Design review of the part built by this model. Coordinates are the model's own, in mm. Face numbers are marked on the shaded views. A direction names the side the tool comes from. Coordinates: 2 decimals unless noted, no trailing zeros. Loops run counter-clockwise (first coordinate to the right, second up) from the corner with the lowest first, then second, coordinate; pieces in that order, holes last. Notation, with made-up numbers: M -21.75,-23.75 L 15.25,-23.75 A29 ccw 15.25,11.25 Z; hole C 88.5,36 d9. An arc over 180 degrees is marked long. One line per item, written item: value.
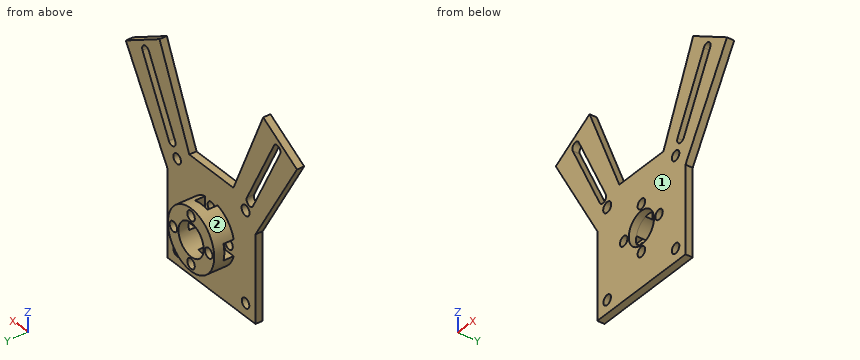
```python
from build123d import *

# Parameters (mm, degrees)
SKETCH_1_R          = 1.7
SKETCH_1_R_2        = 1.8
SKETCH_1_R_3        = 5.7
EXTRUDE_1_DEPTH     = 2.5
SKETCH_2_R          = 10.5
EXTRUDE_2_DEPTH     = 7
SKETCH_4_R          = 1.7
CUT_EXTRUDE_1_DEPTH = 7
CUT_EXTRUDE_2_DEPTH = 3.5
SKETCH_6_R          = 5.7
CUT_EXTRUDE_3_DEPTH = 20


with BuildPart() as part:
    # 草图1 → 凸台-拉伸1 (new body)
    with BuildSketch(Plane(origin=(0, 0, 0), x_dir=(1, 0, 0), z_dir=(0, 1, 0))):
        Polygon((-9.99944515, -20.000324527), (10.00055485, -20.000324527), (23.493176713, -51.085714784), (38.795982487, -42.134997854), (20, -10), (20, 20), (-20, 20), (-20, -10), (-38.79573581, -42.1354119), (-23.493239928, -51.085714784), align=None)
        with Locations((15.5, 15.5)):
            Circle(SKETCH_1_R, mode=Mode.SUBTRACT)
        with Locations((-15.5, -15.5)):
            Circle(SKETCH_1_R_2, mode=Mode.SUBTRACT)
        with Locations((-15.5, 15.5)):
            Circle(SKETCH_1_R, mode=Mode.SUBTRACT)
        Circle(SKETCH_1_R_3, mode=Mode.SUBTRACT)
        with Locations((-8, 0)):
            Circle(SKETCH_1_R, mode=Mode.SUBTRACT)
        with Locations((0, 8)):
            Circle(SKETCH_1_R, mode=Mode.SUBTRACT)
        with Locations((8, 0)):
            Circle(SKETCH_1_R, mode=Mode.SUBTRACT)
        with Locations((0, -8)):
            Circle(SKETCH_1_R, mode=Mode.SUBTRACT)
        with Locations((15.5, -15.5)):
            Circle(SKETCH_1_R, mode=Mode.SUBTRACT)
        with BuildLine():
            Line((-16.131862345, -20.121977189), (-28.419219954, -44.445930008))
            ThreePointArc((-28.419219954, -44.445930008), (-30.461319047, -45.117305053), (-31.132694091, -43.07520596))
            Line((-31.132694091, -43.07520596), (-18.845336482, -18.75125314))
            ThreePointArc((-18.845336482, -18.75125314), (-16.803237389, -18.079878096), (-16.131862345, -20.121977189))
        make_face(mode=Mode.SUBTRACT)
        with BuildLine():
            Line((19.251434516, -19.436615165), (31.203359651, -43.037711333))
            ThreePointArc((31.203359651, -43.037711333), (30.498813674, -45.187970612), (28.348554395, -44.483424635))
            Line((28.348554395, -44.483424635), (16.39662926, -20.882328467))
            ThreePointArc((16.39662926, -20.882328467), (17.101175237, -18.732069188), (19.251434516, -19.436615165))
        make_face(mode=Mode.SUBTRACT)
    extrude(amount=EXTRUDE_1_DEPTH)

    # 草图2 → 凸台-拉伸2 (add)
    with BuildSketch(Plane(origin=(0, 2.5, 0), x_dir=(1, 0, 0), z_dir=(0, 1, 0))):
        Circle(SKETCH_2_R)
    extrude(amount=EXTRUDE_2_DEPTH)

    # 草图4 → 切除-拉伸1 (cut)
    with BuildSketch(Plane.XZ.offset(-2.5)):
        with Locations((0, -8)):
            Circle(SKETCH_4_R)
        with Locations((-8, 0)):
            Circle(SKETCH_4_R)
        with Locations((8, 0)):
            Circle(SKETCH_4_R)
        with Locations((0, 8)):
            Circle(SKETCH_4_R)
    extrude(amount=-CUT_EXTRUDE_1_DEPTH, mode=Mode.SUBTRACT)

    # 草图5 → 切除-拉伸2 (cut)
    with BuildSketch(Plane(origin=(0, 2.5, 0), x_dir=(1, 0, 0), z_dir=(0, 1, 0))):
        Polygon((-4.766838493, 0), (-6.383419246, 2.8), (-11.233161507, 2.8), (-11.233161507, -2.8), (-6.383419246, -2.8), align=None)
        Polygon((4.766838493, 0), (6.383419246, -2.8), (11.233161507, -2.8), (11.233161507, 2.8), (6.383419246, 2.8), align=None)
        Polygon((-2.8, 11.233161507), (-2.8, 6.383419246), (0, 4.766838493), (2.8, 6.383419246), (2.8, 11.233161507), align=None)
        Polygon((0, -4.766838493), (-2.8, -6.383419246), (-2.8, -11.233161507), (2.8, -11.233161507), (2.8, -6.383419246), align=None)
    extrude(amount=CUT_EXTRUDE_2_DEPTH, mode=Mode.SUBTRACT)

    # 草图6 → 切除-拉伸3 (cut)
    with BuildSketch(Plane.XZ.offset(-2.5)):
        Circle(SKETCH_6_R)
    extrude(amount=-CUT_EXTRUDE_3_DEPTH, mode=Mode.SUBTRACT)


solid = part.part
```
(1) Insertion check: pin 1 (1 mm diameter, centred on x = 8.5, y = 3.5, fed in from -Z); pin 2 (1 mm diameter, centred on y = 8.5, z = 6.5, fed in from +X); pin 3 (1.2 mm diameter, centred on x = 4.5, y = 1.5, fed in from +Z). Each pin has a flat end and moves straight along its axis. Give the tip position at first contact, or say it passes through.
Reply:
pin 1: stops at z = -6.8
pin 2: stops at x = 8.62
pin 3: stops at z = 20
(2) We need section C-C on z = -15.5. State the section outline as (x, y) points.
Reply:
outline: M -20,0 L -17.2,0 L -17.2,2.5 L -20,2.5 Z; M -13.8,0 L 13.8,0 L 13.8,2.5 L -13.8,2.5 Z; M 17.2,0 L 20,0 L 20,2.5 L 17.2,2.5 Z
(3) We need section B-B on y = 3.75. State the section outline as (x, z) points.
Reply:
outline: M -10.12,-2.8 A10.5 ccw -2.8,-10.12 L -2.8,-6.38 L -1.34,-5.54 A5.7 cw -5.54,-1.34 L -6.38,-2.8 Z; M -10.12,2.8 L -6.38,2.8 L -5.54,1.34 A5.7 cw -1.34,5.54 L -2.8,6.38 L -2.8,10.12 A10.5 ccw Z; M 1.34,-5.54 L 2.8,-6.38 L 2.8,-10.12 A10.5 ccw 10.12,-2.8 L 6.38,-2.8 L 5.54,-1.34 A5.7 cw Z; M 1.34,5.54 A5.7 cw 5.54,1.34 L 6.38,2.8 L 10.12,2.8 A10.5 ccw 2.8,10.12 L 2.8,6.38 Z
(4) We need section A-A on x = 0. State how many separate pieces and enclosed holes the cut face has, then the cut area to 3 significant figures.
Reply:
separate pieces: 8
enclosed holes: 0
area: 64.3 mm2
(5) To check wall thickness, follow line 1 along X through (y, z) = (1.9, -15.5); line 2 along Z through (x, y) = (0, 1.45); line 3 along X through (y, z) = (1.5, 25). State the ranges of each line that lie inside material, in increasing order. Write a range as [from, to].
Reply:
line 1: x = [-20, -17.2], [-13.8, 13.8], [17.2, 20]
line 2: z = [-20, -9.7], [-6.3, -5.7], [5.7, 6.3], [9.7, 20]
line 3: x = [-28.77, -22], [-18.6, -12.17], [12.17, 18.48], [22.07, 28.77]
(6) We need section D-D on z = -8. State the section outline as (x, y) points.
Reply:
outline: M -20,0 L -1.7,0 L -1.7,2.5 L -2.8,2.5 L -2.8,6 L -1.7,6 L -1.7,9.5 L -6.8,9.5 L -6.8,2.5 L -20,2.5 Z; M 1.7,0 L 20,0 L 20,2.5 L 6.8,2.5 L 6.8,9.5 L 1.7,9.5 L 1.7,6 L 2.8,6 L 2.8,2.5 L 1.7,2.5 Z
(7) Tool access review of the marked faces 1 and 2: name each direction out of +Z, -Z, +X, -X, +Y, -Y from which nothing blocks a thin tool from reaching the whole face with its end or side.
Reply:
face 1: +Z, -Z, +X, -X, -Y
face 2: +Y
